Design review of the part built by this model. Coordinates are the model's own, in mm. A direction names the side the tool comes from. Coordinates: 2 decimals unless noted, no trailing zeros. Write each loop counter-clockwise with the first axis right and the second up, starting at its lowest first coordinate (ties: lowest second). Pieces come first, ordered by that corner, then holes. Notation, with made-up numbers: (-33.5, 76.5) -> (25.5, 76.5) arc R26 cw to (25.5, 97.5) -> close; hole circle Ø4 at (51, 67). An arc over 180 degrees is marked (long way). Return JSON: item names as keys, results as strings. Group by question number.
from build123d import *

# Parameters (mm, degrees)
SKETCH1_W                  = 47.5
SKETCH1_H                  = 110
SKETCH1_R                  = 2
SKETCH1_W_2                = 10
SKETCH1_H_2                = 10
BOSS_EXTRUDE1_DEPTH        = 4
SKETCH2_R                  = 12.5
SKETCH2_R_2                = 7.5
BOSS_EXTRUDE2_DEPTH        = 30
SKETCH4_R                  = 12.5
SKETCH4_R_2                = 7.5
BOSS_EXTRUDE3_DEPTH        = 60
SZKIC1_W                   = 47.5
SZKIC1_H                   = 5.522276491
WYTNIJ_WYCI_GNI_CIE1_DEPTH = 10.5
SZYK_LINIOWY1_COUNT        = 2
SZYK_LINIOWY1_PITCH        = 50


with BuildPart() as part:
    # Sketch1 → Boss-Extrude1 (new body)
    with BuildSketch(Plane(origin=(0, 0, 0), x_dir=(1, 0, 0), z_dir=(0, 1, 0))):
        with Locations((-12.897727273, -28.125)):
            Rectangle(SKETCH1_W, SKETCH1_H)
        with Locations(Location((0.852272727, 17.315, 0), (0, 0, 270))):
            Circle(SKETCH1_R, mode=Mode.SUBTRACT)
        with Locations(Location((-29.147727273, -8.845, 0), (0, 0, 270))):
            Circle(SKETCH1_R, mode=Mode.SUBTRACT)
        with Locations(Location((0.852272727, -45.685, 0), (0, 0, 270))):
            Circle(SKETCH1_R, mode=Mode.SUBTRACT)
        with Locations(Location((0.852272727, -74.045, 0), (0, 0, 270))):
            Circle(SKETCH1_R, mode=Mode.SUBTRACT)
        with Locations(Location((-29.147727273, -74.045, 0), (0, 0, 270))):
            Circle(SKETCH1_R, mode=Mode.SUBTRACT)
        with Locations((-14.147727273, 1.875)):
            Rectangle(SKETCH1_W_2, SKETCH1_H_2, mode=Mode.SUBTRACT)
        with Locations((-14.147727273, -48.125)):
            Rectangle(SKETCH1_W_2, SKETCH1_H_2, mode=Mode.SUBTRACT)
    extrude(amount=-BOSS_EXTRUDE1_DEPTH)

    # Sketch2 → Boss-Extrude2 (add)
    with BuildSketch(Plane(origin=(0, 0, 0), x_dir=(1, 0, 0), z_dir=(0, 1, 0))):
        with Locations(Location((-14.147727273, -48.125, 0), (0, 0, 270))):
            Circle(SKETCH2_R)
        with Locations(Location((-14.147727273, -48.125, 0), (0, 0, 270))):
            Circle(SKETCH2_R_2, mode=Mode.SUBTRACT)
    extrude(amount=BOSS_EXTRUDE2_DEPTH)

    # Sketch4 → Boss-Extrude3 (add)
    with BuildSketch(Plane(origin=(0, 0, 0), x_dir=(1, 0, 0), z_dir=(0, 1, 0))):
        with Locations(Location((-14.147727273, 1.875, 0), (0, 0, 270))):
            Circle(SKETCH4_R)
        with Locations(Location((-14.147727273, 1.875, 0), (0, 0, 270))):
            Circle(SKETCH4_R_2, mode=Mode.SUBTRACT)
    extrude(amount=BOSS_EXTRUDE3_DEPTH)

    # Szkic1 → Wytnij-wyciągnięcie1 (cut)
    with BuildSketch(Plane(origin=(0, 0, 0), x_dir=(1, 0, 0), z_dir=(0, 1, 0))):
        with Locations((-12.897727273, -80.363861754)):
            Rectangle(SZKIC1_W, SZKIC1_H)
    extrude(amount=-WYTNIJ_WYCI_GNI_CIE1_DEPTH, mode=Mode.SUBTRACT)

    # Szkic3 → Wycięcie-obrót1 (revolve, cut)
    with BuildSketch(Plane(origin=(-30.053799947, 0, 14.014317072), x_dir=(-0.4226182617407009, 0, -0.9063077870366493), z_dir=(0.9063077870366493, 0, -0.4226182617407009)), mode=Mode.PRIVATE) as wyci_cie_obr_t1_sk:
        Polygon((-31.038274345, 24.733727238), (-30.433976709, 26.129177698), (-29.168033578, 25.580963009), (-28.580169258, 26.938465486), (-22.156612406, 24.156754256), (-23.348774361, 21.40380132), align=None)
    wyci_cie_obr_t1 = revolve(wyci_cie_obr_t1_sk.sketch.rotate(Axis((-15.574618004, 26.129177698, 45.065022951), (-0.3878160615913765, -0.3973873185023342, -0.8316742279674645)), 190.498100282), axis=Axis((-15.574618004, 26.129177698, 45.065022951), (-0.3878160615913765, -0.3973873185023342, -0.8316742279674645)), mode=Mode.SUBTRACT)

    # Szyk liniowy1: Wycięcie-obrót1 ×2
    with Locations(*[(0, 0, -i * SZYK_LINIOWY1_PITCH) for i in range(1, SZYK_LINIOWY1_COUNT)]):
        add(wyci_cie_obr_t1, mode=Mode.SUBTRACT)


solid = part.part
Q1. For P1, Ø6, axis at x = 4, z = -3.5, coming from the +Y side; P2, Ø5, axis at x = -8.5, y = 45.5, coming from the +Z side; P3, Ø1.5, axis at x = -9.5, y = 20, coming from the +Z side, all flat-tipped, find the tip position at first contact; note any pin that passes through.
Q2. We need section D-D on x = -24. Write out the cut boundary in (y, z) (3 decimals).
Q3. We need section A-A on z = 46. Write out the cut boundary in (x, y), plus the area to 3 significant figures.
Q4. We need section B-B on z = 9.5. Write out the cut boundary in (x, y).
Q5. Wall thickness on L1, parallel to Z at x = -17.5, y = 2; L2, parallel to Y at x = 2.5, z = 7.5; L3, parallel to X at y = 14, z = 52.5: over which ranges is each line inside the solid? List them lowest first.
Q6. For faces 4 (the flat face through (-17.51, 26.075, 40.113)), 5 (the flat face through (-9.148, -2, -2)), 6 (the cylindrical face through (-11.895, 29.58, 5.279)), list the 3-axis set-ups (+Z, -Z, +X, -X, +Y, -Y) from which the entire face can be reached by the end or side of a thin tool; tool diameter is ignored.
Q7. We need section C-C on y = 11. Write out the cut boundary in (x, z) (3 decimals), plus the area to 3 significant figures.
Q8. The part is to be moulded in two halves that separate along X. For faces 1 (the flat face through (-13, -2, 77.603)), 2 (the cylindrical face through (1.453, -1.972, 75.953)), 3 (the flat face through (10.852, -2, 26)), say which applies: +X half, -X half, draft (parallel to the pull), parting line (faces both ways), or undercut.
Findings below:
{
 "1": {"P1": "stops at y = 0", "P2": "stops at z = 10.22", "P3": "stops at z = 60"},
 "2": {"outline": "(-4, -26.875) -> (0, -26.875) -> (0, -9.568) -> (60, -9.568) -> (60, 5.818) -> (0, 5.818) -> (0, 40.432) -> (30, 40.432) -> (30, 55.818) -> (0, 55.818) -> (0, 77.603) -> (-4, 77.603) -> close"},
 "3": {"outline": "(-36.65, -4) -> (-19.15, -4) -> (-19.15, 0) -> (-21.34, 0) -> (-21.34, 30) -> (-26.47, 30) -> (-26.47, 0) -> (-36.65, 0) -> close; (-9.15, -4) -> (-1.12, -4) -> (-1.12, 0) -> (-1.83, 0) -> (-1.83, 30) -> (-6.96, 30) -> (-6.96, 0) -> (-9.15, 0) -> close; (2.83, -4) -> (10.85, -4) -> (10.85, 0) -> (2.83, 0) -> close", "area": "442 mm^2"},
 "4": {"outline": "(-36.65, -4) -> (-31.04, -4) -> (-31.04, 0) -> (-36.65, 0) -> close; (-27.26, -4) -> (10.85, -4) -> (10.85, 0) -> (-8.97, 0) -> (-8.97, 60) -> (-19.33, 60) -> (-19.33, 0) -> (-27.26, 0) -> close"},
 "5": {"L1": "z = -13.92 to -8.58, 4.83 to 10.17, 36.08 to 41.42, 54.83 to 60.17", "L2": "y = -4 to 0", "L3": "x = -25.86 to -20.24, -8.06 to -2.44"},
 "6": {"face 4": "none", "face 5": "+Y, -Y", "face 6": "+Y"},
 "7": {"outline": "circle Ø25 at (-14.148, -1.875); circle Ø25 at (-14.148, 48.125); hole circle Ø15 at (-14.148, -1.875); hole circle Ø15 at (-14.148, 48.125)", "area": "628 mm^2"},
 "8": {"face 1": "draft", "face 2": "undercut", "face 3": "+X half"}
}
